Job drawing, mm, ordinate dimensions from the low corner. One solid piece. A direction names the side the tool comes from. Coordinates: 2 decimals unless noted, no trailing zeros. Write each loop counter-clockwise with the first axis right and the second up, starting at its lowest first coordinate (ties: lowest second). Pieces come first, ordered by that corner, then holes. Notation, with made-up numbers: (37.5, -28) -> (64.5, -28) arc R3 ccw to (64.5, -23) -> close; hole circle Ø9 at (-34.5, 14). An arc over 180 degrees is marked (long way). One line per question, with ' | ' between items. Start each with the question number.
Item 1: Saw through at B-B (z = 18.5). List the corners of the cut face in (x, y) (1 decimal), and give its area (3 significant figures).
Item 2: Probe probe 1 along Z at (x, y) = (14.5, 3); probe 2 along Y at (x, z) = (50.65, 8); probe 3 along Y at (x, z) = (47, 8). List the from-to ranges inside material, lowest first. Write a range as [from, to].
Item 3: Pin check, flat tips, straight feed: pin 1 (6 mm diameter, centred on y = 25, z = 31, fed in from -X) (3 decimals); pin 2 (5 mm diameter, centred on y = 28, z = 42.5, fed in from +X) (3 decimals); pin 3 (10 mm diameter, centred on x = 31.5, z = 44.5, fed in from +Y). Stop position of each tip, or through.
Item 4: Two-plate mould, pull along X, no slides. Class the marked faces 1, 2, 3 and 4: pulls with the +X half, pulls with the -X half, needs draft (parallel to the pull), parting line crosses it, or undercut.
Item 5: Saw through at A-A (y = 20.5). List the corners of the cut face in (x, z) (1 decimal), and give its area (3 significant figures).
Item 6: Saw through at C-C (y = 15). List the corners of the cut face in (x, z) (1 decimal).
Item 7: 3-axis set-ups, long thin cutter, end or side, ignore diameter. For the marked faces 5, 6, 7, 8 and 9: which of +Z, -Z, +X, -X, +Y, -Y reach the whole face in a straight line?
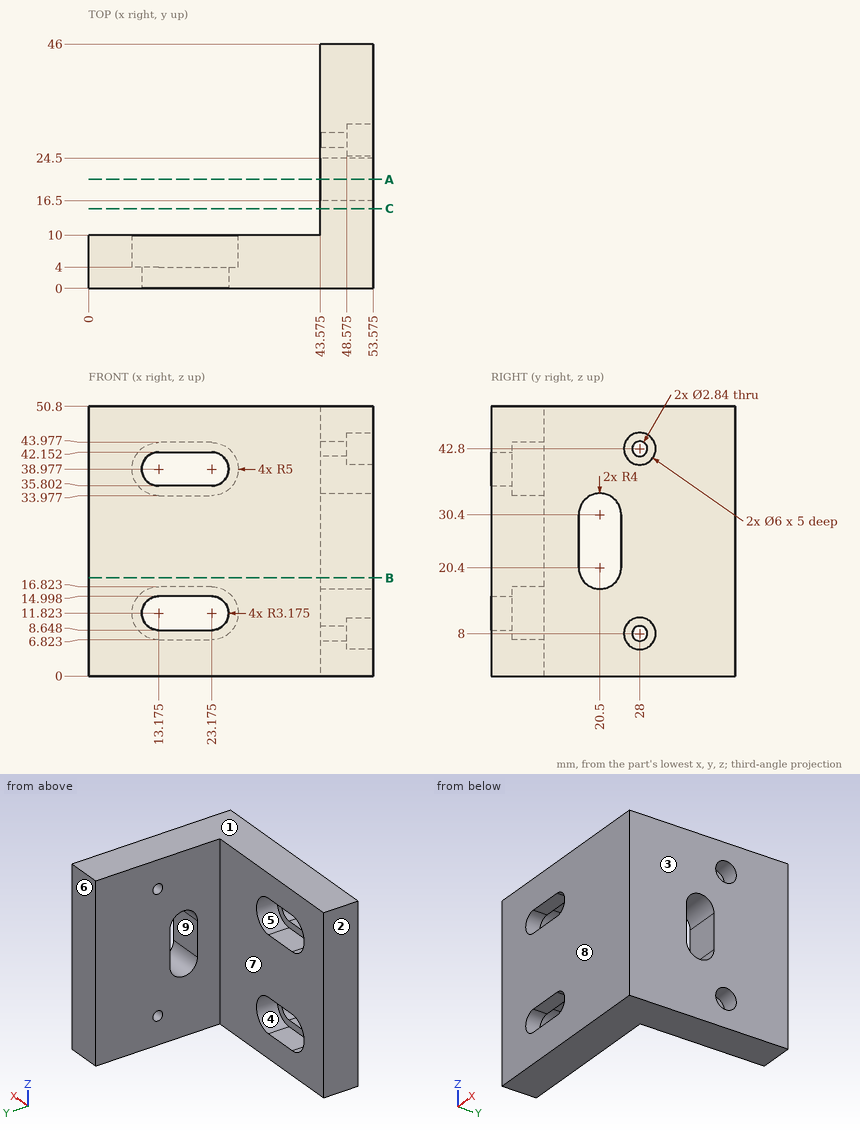
From the geometry:
1) outline: (0, 0) -> (53.6, 0) -> (53.6, 17) -> (43.6, 17) -> (43.6, 10) -> (0, 10) -> close; (43.6, 24) -> (53.6, 24) -> (53.6, 46) -> (43.6, 46) -> close | area: 825 mm2
2) probe 1: [0, 8.65], [15, 35.8], [42.15, 50.8] | probe 2: [0, 25], [31, 46] | probe 3: [0, 26.58], [29.42, 46]
3) pin 1: x = 43.575 | pin 2: x = 48.575 | pin 3: y = 10
4) face 1: needs draft | face 2: pulls with the -X half | face 3: pulls with the +X half | face 4: undercut
5) outline: (43.6, 0) -> (53.6, 0) -> (53.6, 16.4) -> (43.6, 16.4) -> close; (43.6, 34.4) -> (53.6, 34.4) -> (53.6, 50.8) -> (43.6, 50.8) -> close | area: 328 mm2
6) outline: (43.6, 0) -> (53.6, 0) -> (53.6, 50.8) -> (43.6, 50.8) -> close
7) face 5: +Y | face 6: +Z, -Z, +X, -X, +Y | face 7: +Z, -Z, -X, +Y | face 8: +Z, -Z, +X, -X, -Y | face 9: +X, -X
